from build123d import *

# Parameters (mm, degrees)
ESQUISSE1_R        = 15
ESQUISSE1_R_2      = 1.6
ESQUISSE1_R_3      = 2.75
BOSS_EXTRU_1_DEPTH = 2
ESQUISSE2_R        = 7
ESQUISSE2_R_2      = 2.75
BOSS_EXTRU_2_DEPTH = 4
ESQUISSE3_R        = 4
ESQUISSE3_R_2      = 2.75
BOSS_EXTRU_3_DEPTH = 2


with BuildPart() as part:
    # Esquisse1 → Boss.-Extru.1 (new body)
    with BuildSketch(Plane.XY):
        Circle(ESQUISSE1_R)
        with Locations((0, 12.5)):
            Circle(ESQUISSE1_R_2, mode=Mode.SUBTRACT)
        with Locations((-10.825317547, 6.25)):
            Circle(ESQUISSE1_R_2, mode=Mode.SUBTRACT)
        with Locations((-10.825317547, -6.25)):
            Circle(ESQUISSE1_R_2, mode=Mode.SUBTRACT)
        with Locations((0, -12.5)):
            Circle(ESQUISSE1_R_2, mode=Mode.SUBTRACT)
        with Locations((10.911920088, -6.3)):
            Circle(ESQUISSE1_R_2, mode=Mode.SUBTRACT)
        with Locations((10.825317547, 6.25)):
            Circle(ESQUISSE1_R_2, mode=Mode.SUBTRACT)
        Circle(ESQUISSE1_R_3, mode=Mode.SUBTRACT)
    extrude(amount=BOSS_EXTRU_1_DEPTH)

    # Esquisse2 → Boss.-Extru.2 (add)
    with BuildSketch(Plane.XY.offset(2)):
        Circle(ESQUISSE2_R)
        Circle(ESQUISSE2_R_2, mode=Mode.SUBTRACT)
    extrude(amount=BOSS_EXTRU_2_DEPTH)

    # Esquisse3 → Boss.-Extru.3 (add)
    with BuildSketch(Plane.XY.offset(6)):
        Circle(ESQUISSE3_R)
        Circle(ESQUISSE3_R_2, mode=Mode.SUBTRACT)
    extrude(amount=BOSS_EXTRU_3_DEPTH)


solid = part.part
Can you work these out from the model? Positions are in its coordinate system, mm. A direction names the side the tool comes from. Coordinates: 2 decimals unless noted, no trailing zeros. Order: outer loops, then holes, each group sorted by start corner. A loop starts at its lowest first (then second) coordinate and runs counter-clockwise, first axis right, second up. Notation, with made-up numbers: M -10,36 L -3,36 A33 ccw -3,73 Z; hole C 31.25,-21.75 d11. An arc over 180 degrees is marked long. Write item = value, one per line.
(1) Suppose I cut it at A-A on x = 0. Please give me the cut outline in (y, z).
Results are:
outline = M -15,0 L -14.1,0 L -14.1,2 L -15,2 Z; M -10.9,0 L -2.75,0 L -2.75,8 L -4,8 L -4,6 L -7,6 L -7,2 L -10.9,2 Z; M 2.75,0 L 10.9,0 L 10.9,2 L 7,2 L 7,6 L 4,6 L 4,8 L 2.75,8 Z; M 14.1,0 L 15,0 L 15,2 L 14.1,2 Z
(2) For pin 1 Ø1 at (x, z) = (4, 5) entering from +Y; pin 2 Ø5 at (x, y) = (0, -12.5) entering from +Z; pin 3 Ø1 at (y, z) = (-7, 2) entering from -X, each with a flat end and sliding along its axis, tell me the tip position at first contact or that it passes through.
Results are:
pin_1 = 6.06
pin_2 = 2
pin_3 = -13.52
(3) Suppose I cut it at C-C on x = -11.5. Please give me the cut outline in (y, z), plus the area to 3 significant figures.
Results are:
outline = M -9.63,0 L -7.7,0 L -7.7,2 L -9.63,2 Z; M -4.8,0 L 4.8,0 L 4.8,2 L -4.8,2 Z; M 7.7,0 L 9.63,0 L 9.63,2 L 7.7,2 Z
area = 26.9 mm2
(4) Suppose I cut it at B-B on y = 0. Please give me the cut outline in (x, z).
Results are:
outline = M -15,0 L -2.75,0 L -2.75,8 L -4,8 L -4,6 L -7,6 L -7,2 L -15,2 Z; M 2.75,0 L 15,0 L 15,2 L 7,2 L 7,6 L 4,6 L 4,8 L 2.75,8 Z
(5) For faces 1 (the face through (-0.35, -14.06, 0.99)), 2 (the face through (6.466, -2.681, 3.972)), which set-ups out of +Z, -Z, +X, -X, +Y, -Y let a thin tool reach every point of the face, with its end or its side?
Results are:
face_1 = +Z, -Z
face_2 = +Z
(6) If we mould it in two halves opening along X, with no side actions, what happens to faces 3 (the face through (-9.347, 5.637, 0.986)), 4 (the face through (-14.985, 0.66, 0.986)), 5 (the face through (3, 0, 0))? For each: pulls with the +X half, pulls with the -X half, needs draft (parallel to the pull), parting line crosses it, or undercut.
Results are:
face_3 = undercut
face_4 = parting line crosses it
face_5 = needs draft
(7) Suppose I cut it at D-D on y = 6.25. Please give me the cut outline in (x, z), plus the area to 3 significant figures.
Results are:
outline = M -13.64,0 L -12.43,0 L -12.43,2 L -13.64,2 Z; M -9.23,0 L 9.23,0 L 9.23,2 L 3.15,2 L 3.15,6 L -3.15,6 L -3.15,2 L -9.23,2 Z; M 12.43,0 L 13.64,0 L 13.64,2 L 12.43,2 Z
area = 67.0 mm2
(8) I need wall thicknesses on line 1 along Y through (x, z) = (0, 1.5); line 2 along Y through (x, z) = (0, 4.25); line 3 along Z through (x, y) = (4.5, 9.5). Which ranges of each line are inside material? Lowest first, please. Write a range as [from, to].
Results are:
line_1 = [-15, -14.1], [-10.9, -2.75], [2.75, 10.9], [14.1, 15]
line_2 = [-7, -2.75], [2.75, 7]
line_3 = [0, 2]
